Here's how the part is built. I have some questions about the finished solid (model axes, mm). A direction names the side the tool comes from. Round coordinates to 2 decimals unless told otherwise and drop trailing zeros. Write each loop counter-clockwise with the first axis right and the second up, starting at its lowest first coordinate (ties: lowest second). Pieces come first, ordered by that corner, then holes. Notation, with made-up numbers: (12.5, 76) -> (38.5, 76) arc R18 cw to (38.5, 110) -> close; hole circle Ø7 at (-20.75, 47). An arc over 180 degrees is marked (long way). Answer in a Markdown table with one row per item.
from build123d import *

# Parameters (mm, degrees)
SKETCH_1_R          = 4
SKETCH_1_R_2        = 1
EXTRUDE_1_DEPTH     = 5
EXTRUDE_START       = -2
SKETCH_2_R          = 12.25
SKETCH_2_R_2        = 4
SKETCH_2_R_3        = 1.25
EXTRUDE_2_DEPTH     = 2
CHAMFER_1_SIZE      = 0.3
SKETCH_3_R          = 3
CUT_EXTRUDE_1_DEPTH = 0.5
SKETCH_4_R          = 2.9
CUT_EXTRUDE_2_DEPTH = 3


with BuildPart() as part:
    # 草图1 → 凸台-拉伸1 (new body)
    with BuildSketch(Plane(origin=(0, 0, 0), x_dir=(1, 0, 0), z_dir=(0, 1, 0))):
        with Locations(Location((0, 0, 0), (0, 0, 270))):
            Circle(SKETCH_1_R)
        with Locations(Location((0, 0, 0), (0, 0, 270))):
            Circle(SKETCH_1_R_2, mode=Mode.SUBTRACT)
    extrude(amount=EXTRUDE_1_DEPTH)

    # 草图2 → 凸台-拉伸2 (add)
    with BuildSketch(Plane(origin=(0, 5, 0), x_dir=(1, 0, 0), z_dir=(0, 1, 0)).offset(EXTRUDE_START)):
        with Locations(Location((0, 0, 0), (0, 0, 270))):
            Circle(SKETCH_2_R)
        with Locations(Location((0, 0, 0), (0, 0, 270))):
            Circle(SKETCH_2_R_2, mode=Mode.SUBTRACT)
        with Locations(Location((0, 8, 0), (0, 0, 270))):
            Circle(SKETCH_2_R_3, mode=Mode.SUBTRACT)
        with Locations(Location((8, 0, 0), (0, 0, 270))):
            Circle(SKETCH_2_R_3, mode=Mode.SUBTRACT)
        with Locations(Location((0, -8, 0), (0, 0, 270))):
            Circle(SKETCH_2_R_3, mode=Mode.SUBTRACT)
        with Locations(Location((-8, 0, 0), (0, 0, 270))):
            Circle(SKETCH_2_R_3, mode=Mode.SUBTRACT)
    extrude(amount=EXTRUDE_2_DEPTH)

    # 倒角1
    chamfer_1_edges = [part.edges().sort_by_distance(p)[0] for p in [
        (0, 3, -12.25),
        (0, 5, -12.25),
        (0, 0, -4),
        (0, 3, -4),
    ]]
    chamfer(chamfer_1_edges, length=CHAMFER_1_SIZE)

    # 草图3 → 切除-拉伸1 (cut)
    with BuildSketch(Plane(origin=(0, 5, 0), x_dir=(1, 0, 0), z_dir=(0, 1, 0))):
        with Locations(Location((0, 0, 0), (0, 0, 270))):
            Circle(SKETCH_3_R)
    extrude(amount=-CUT_EXTRUDE_1_DEPTH, mode=Mode.SUBTRACT)

    # 草图4 → 切除-拉伸2 (cut)
    with BuildSketch(Plane.XZ):
        with Locations(Location((0, 0, 0), (0, 0, 270))):
            Circle(SKETCH_4_R)
    extrude(amount=-CUT_EXTRUDE_2_DEPTH, mode=Mode.SUBTRACT)


solid = part.part
1) I want a section at A-A, the plane x = 0. Count the separate pieces of the cut face and the enclosed holes in it, and give its area (3 significant figures).
Response:
| item | result |
|---|---|
| separate pieces | 4 |
| enclosed holes | 0 |
| area | 39.4 mm^2 |
2) I need wall thicknesses on line 1 (X direction, y = 4.15, z = 0); line 2 (X direction, y = 4.85, z = 0); line 3 (Y direction, x = 6, z = -6.25). Which ranges of each line are inside material? Lowest first, please. Write a range as [from, to].
Response:
| item | result |
|---|---|
| line 1 | x = [-12.25, -9.25], [-6.75, -1], [1, 6.75], [9.25, 12.25] |
| line 2 | x = [-12.1, -9.25], [-6.75, -3], [3, 6.75], [9.25, 12.1] |
| line 3 | y = [3, 5] |
3) Which directions (+Z, -Z, +X, -X, +Y, -Y) give clear straight access to the entire face, cutting with the end or side of a thin tool? Please do faces 1 (the face through (-2.5, 5, 2.5)), 2 (the face through (1, 4.5, -1)), 3 (the face through (0, 3, -1.2)).
Response:
| item | result |
|---|---|
| face 1 | +Z, -Z, +X, -X, +Y |
| face 2 | +Y |
| face 3 | -Y |
4) I want a section at C-C, the plane y = 0.7. List the corners of the cut face in (x, z) for me.
Response:
| item | result |
|---|---|
| outline | circle Ø8 at (0, 0); hole circle Ø5.8 at (0, 0) |
5) For pin 1 (3 mm diameter, centred on x = 2, z = -6.5, fed in from -Y); pin 2 (1.5 mm diameter, centred on x = 1.5, y = 2, fed in from -Z); pin 3 (2 mm diameter, centred on x = -9.5, y = 4, fed in from -Z); pin 4 (2 mm diameter, centred on x = 0, z = 8, fed in from -Y), each with a flat end and sliding along its axis, tell me the tip position at first contact or that it passes through.
Response:
| item | result |
|---|---|
| pin 1 | stops at y = 3 |
| pin 2 | stops at z = -3.93 |
| pin 3 | stops at z = -8.82 |
| pin 4 | passes through |
